Check sheet for the modelled part. Datum: model origin and axes. Units: mm. A direction names the side the tool comes from. Give positions to 0.01 mm unless a question says otherwise; leave off trailing zeros. Loops run counter-clockwise (first coordinate to the right, second up) from the corner with the lowest first, then second, coordinate; pieces in that order, holes last. Notation, with made-up numbers: (7.25, 37.25) - (65.25, 37.25) arc R27 cw to (65.25, 56.25) - close; hole circle Ø11 at (-10.5, 52). An arc over 180 degrees is marked (long way). Answer in a Markdown table with one row per item. Add a question column.
(1) Sectioned sample at B-B on y = 2.5. Enter the section's corners in (x, z), then the cut area to 3 significant figures.
(2) Sectioned sample at C-C on x = 15.5. Enter the section's corners in (y, z).
(3) Go/stop test with flat-tipped pins: P1, Ø5.5, axis at x = 15.5, z = -15.5, coming from the -Y side; P2, Ø19, axis at x = 0, z = 0, coming from the +Y side; P3, Ø3, axis at x = -2, z = -1, coming from the +Y side. Record where each tip stops, or that it passes through.
(4) Draft check along X on faces 4 (the face through (-19.122, 4.549, 19.061)), 5 (the face through (0, 4, 21.15)), 6 (the face through (-2.736, 1.014, 10.213)). Enter one of: released by +X, released by -X, zero draft, split by the parting line, or undercut.
(5) Sectioned sample at A-A on x = 0. Enter the section's corners in (y, z).
(6) Thickness scan on L1, parallel to Z at x = 0, y = 1.2; L2, parallel to Y at x = 14.5, z = 11.5; L3, parallel to Y at x = 3, z = -3.5. Record the ranges inside material, lowest first.
(7) Sectioned sample at D-D on z = 15.5. Enter the section's corners in (x, y).
(8) Set-up check for faces 1 (the face through (3.3, 1, -0.1)), 2 (the face through (11.42, 10.25, 11.42)), 3 (the face through (2.736, 1.014, -10.213)): record each of +Z, -Z, +X, -X, +Y, -Y from which the full face is reachable in a straight line by a thin tool's end or side.
from build123d import *

# Parameters (mm, degrees)
SKETCH2_W           = 42.3
SKETCH2_H           = 42.3
BOSS_EXTRUDE1_DEPTH = 8
SKETCH5_R           = 29.910616844
SKETCH5_R_2         = 27
CUT_EXTRUDE4_DEPTH  = 9
SKETCH6_R           = 16
CUT_EXTRUDE7_DEPTH  = 7
SKETCH8_R           = 16
SKETCH8_R_2         = 5.1
BOSS_EXTRUDE3_DEPTH = 1
CUT_EXTRUDE8_DEPTH  = 3
FILLET1_R           = 1
SKETCH10_R          = 3
CUT_EXTRUDE9_DEPTH  = 2
SKETCH7_R           = 1.75
CUT_EXTRUDE6_DEPTH  = 9
CHAMFER4_SIZE       = 1
CHAMFER5_SIZE       = 2
CHAMFER6_SIZE       = 0.5
SKETCH11_R          = 17.25
SKETCH11_R_2        = 16
BOSS_EXTRUDE4_DEPTH = 2.25


with BuildPart() as part:
    # Sketch2 → Boss-Extrude1 (new body)
    with BuildSketch(Plane(origin=(0, 0, 0), x_dir=(1, 0, 0), z_dir=(0, 1, 0))):
        Rectangle(SKETCH2_W, SKETCH2_H)
    extrude(amount=BOSS_EXTRUDE1_DEPTH)

    # Sketch5 → Cut-Extrude4 (cut, through all)
    with BuildSketch(Plane(origin=(0, 8, 0), x_dir=(1, 0, 0), z_dir=(0, 1, 0))):
        Circle(SKETCH5_R)
        Circle(SKETCH5_R_2, mode=Mode.SUBTRACT)
    extrude(amount=-CUT_EXTRUDE4_DEPTH, mode=Mode.SUBTRACT)

    # Sketch6 → Cut-Extrude7 (cut)
    with BuildSketch(Plane(origin=(0, 8, 0), x_dir=(1, 0, 0), z_dir=(0, 1, 0))):
        Circle(SKETCH6_R)
    extrude(amount=-CUT_EXTRUDE7_DEPTH, mode=Mode.SUBTRACT)

    # Sketch8 → Boss-Extrude3 (add)
    with BuildSketch(Plane(origin=(0, 1, 0), x_dir=(1, 0, 0), z_dir=(0, 1, 0))):
        Circle(SKETCH8_R)
        Circle(SKETCH8_R_2, mode=Mode.SUBTRACT)
    extrude(amount=BOSS_EXTRUDE3_DEPTH)

    # Sketch9 → Cut-Extrude8 (cut, through all)
    with BuildSketch(Plane(origin=(0, 2, 0), x_dir=(1, 0, 0), z_dir=(0, 1, 0))):
        with BuildLine():
            Line((3.390529491, 12.653628324), (2.096434265, 7.823999193))
            ThreePointArc((2.096434265, 7.823999193), (8.1, 0), (2.096434265, -7.823999193))
            Line((2.096434265, -7.823999193), (3.390529491, -12.653628324))
            ThreePointArc((3.390529491, -12.653628324), (13.1, 0), (3.390529491, 12.653628324))
        make_face()
        with BuildLine():
            Line((-3.390529491, -12.653628324), (-2.096434265, -7.823999193))
            ThreePointArc((-2.096434265, -7.823999193), (-8.1, 0), (-2.096434265, 7.823999193))
            Line((-2.096434265, 7.823999193), (-3.390529491, 12.653628324))
            ThreePointArc((-3.390529491, 12.653628324), (-13.1, 0), (-3.390529491, -12.653628324))
        make_face()
    extrude(amount=-CUT_EXTRUDE8_DEPTH, mode=Mode.SUBTRACT)

    # Fillet1
    fillet1_edges = [part.edges().sort_by_distance(p)[0] for p in [
        (3.390529491, 1, -12.653628324),
        (3.390529491, 1, 12.653628324),
        (2.096434265, 1, 7.823999193),
        (2.096434265, 1, -7.823999193),
        (-2.096434265, 1, -7.823999193),
        (-2.096434265, 1, 7.823999193),
        (-3.390529491, 1, 12.653628324),
        (-3.390529491, 1, -12.653628324),
    ]]
    fillet(fillet1_edges, radius=FILLET1_R)

    # Sketch10 → Cut-Extrude9 (cut, through all)
    with BuildSketch(Plane(origin=(0, 1, 0), x_dir=(1, 0, 0), z_dir=(0, 1, 0))):
        Circle(SKETCH10_R)
    extrude(amount=-CUT_EXTRUDE9_DEPTH, mode=Mode.SUBTRACT)

    # Sketch7 → Cut-Extrude6 (cut, through all)
    with BuildSketch(Plane(origin=(0, 8, 0), x_dir=(1, 0, 0), z_dir=(0, 1, 0))):
        with Locations((-15.5, 15.5)):
            Circle(SKETCH7_R)
        with Locations((15.5, 15.5)):
            Circle(SKETCH7_R)
        with Locations((15.5, -15.5)):
            Circle(SKETCH7_R)
        with Locations((-15.5, -15.5)):
            Circle(SKETCH7_R)
    extrude(amount=-CUT_EXTRUDE6_DEPTH, mode=Mode.SUBTRACT)

    # Chamfer4
    chamfer4_edges = [part.edges().sort_by_distance(p)[0] for p in [
        (21.15, 0, 0),
        (0, 0, 21.15),
        (-21.15, 0, 0),
        (0, 0, -21.15),
        (-19.091883092, 0, 19.091883092),
        (-19.091883092, 0, -19.091883092),
        (19.091883092, 0, -19.091883092),
        (19.091883092, 0, 19.091883092),
    ]]
    chamfer(chamfer4_edges, length=CHAMFER4_SIZE)

    # Chamfer5
    chamfer5_edges = [part.edges().sort_by_distance(p)[0] for p in [
        (-17.25, 0, 15.5),
        (13.75, 0, 15.5),
        (13.75, 0, -15.5),
        (-17.25, 0, -15.5),
    ]]
    chamfer(chamfer5_edges, length=CHAMFER5_SIZE)

    # Chamfer6
    chamfer6_edges = [part.edges().sort_by_distance(p)[0] for p in [
        (-5.1, 2, 0),
    ]]
    chamfer(chamfer6_edges, length=CHAMFER6_SIZE)

    # Sketch11 → Boss-Extrude4 (add)
    with BuildSketch(Plane(origin=(0, 8, 0), x_dir=(1, 0, 0), z_dir=(0, 1, 0))):
        Circle(SKETCH11_R)
        Circle(SKETCH11_R_2, mode=Mode.SUBTRACT)
    extrude(amount=BOSS_EXTRUDE4_DEPTH)


solid = part.part
Reply:
| question | item | result |
|---|---|---|
| 1 | outline | (-21.15, -16.78) arc R27 ccw to (-16.78, -21.15) - (16.78, -21.15) arc R27 ccw to (21.15, -16.78) - (21.15, 16.78) arc R27 ccw to (16.78, 21.15) - (-16.78, 21.15) arc R27 ccw to (-21.15, 16.78) - close; hole circle Ø3.5 at (-15.5, -15.5); hole circle Ø3.5 at (-15.5, 15.5); hole circle Ø32 at (0, 0); hole circle Ø3.5 at (15.5, -15.5); hole circle Ø3.5 at (15.5, 15.5) |
| 1 | area | 911 mm^2 |
| 2 | outline | (0, -20.15) - (1, -21.15) - (8, -21.15) - (8, -17.25) - (2, -17.25) - (0, -19.25) - close; (0, -11.75) - (2, -13.75) - (8, -13.75) - (8, -7.57) - (10.25, -7.57) - (10.25, -3.97) - (2, -3.97) - (2, 3.97) - (10.25, 3.97) - (10.25, 7.57) - (8, 7.57) - (8, 13.75) - (2, 13.75) - (0, 11.75) - close; (0, 19.25) - (2, 17.25) - (8, 17.25) - (8, 21.15) - (1, 21.15) - (0, 20.15) - close |
| 3 | P1 | y = 1 |
| 3 | P2 | y = 2 |
| 3 | P3 | y = 1 |
| 4 | face 4 | released by -X |
| 4 | face 5 | zero draft |
| 4 | face 6 | undercut |
| 5 | outline | (0, -20.15) - (1, -21.15) - (8, -21.15) - (8, -17.25) - (10.25, -17.25) - (10.25, -16) - (2, -16) - (2, -5.6) - (1.5, -5.1) - (1, -5.1) - (1, -3) - (0, -3) - close; (0, 3) - (1, 3) - (1, 5.1) - (1.5, 5.1) - (2, 5.6) - (2, 16) - (10.25, 16) - (10.25, 17.25) - (8, 17.25) - (8, 21.15) - (1, 21.15) - (0, 20.15) - close |
| 6 | L1 | -21.15 to -5.1, 5.1 to 21.15 |
| 6 | L2 | 0 to 8 |
| 6 | L3 | 0 to 1 |
| 7 | outline | (-21.15, 1) - (-20.15, 0) - (-19.25, 0) - (-17.25, 2) - (-17.25, 8) - (-21.15, 8) - close; (-13.75, 2) - (-11.75, 0) - (11.75, 0) - (13.75, 2) - (13.75, 8) - (7.57, 8) - (7.57, 10.25) - (3.97, 10.25) - (3.97, 2) - (-3.97, 2) - (-3.97, 10.25) - (-7.57, 10.25) - (-7.57, 8) - (-13.75, 8) - close; (17.25, 2) - (19.25, 0) - (20.15, 0) - (21.15, 1) - (21.15, 8) - (17.25, 8) - close |
| 8 | face 1 | +Y |
| 8 | face 2 | +Z, -Z, +X, -X, +Y |
| 8 | face 3 | +Y, -Y |
